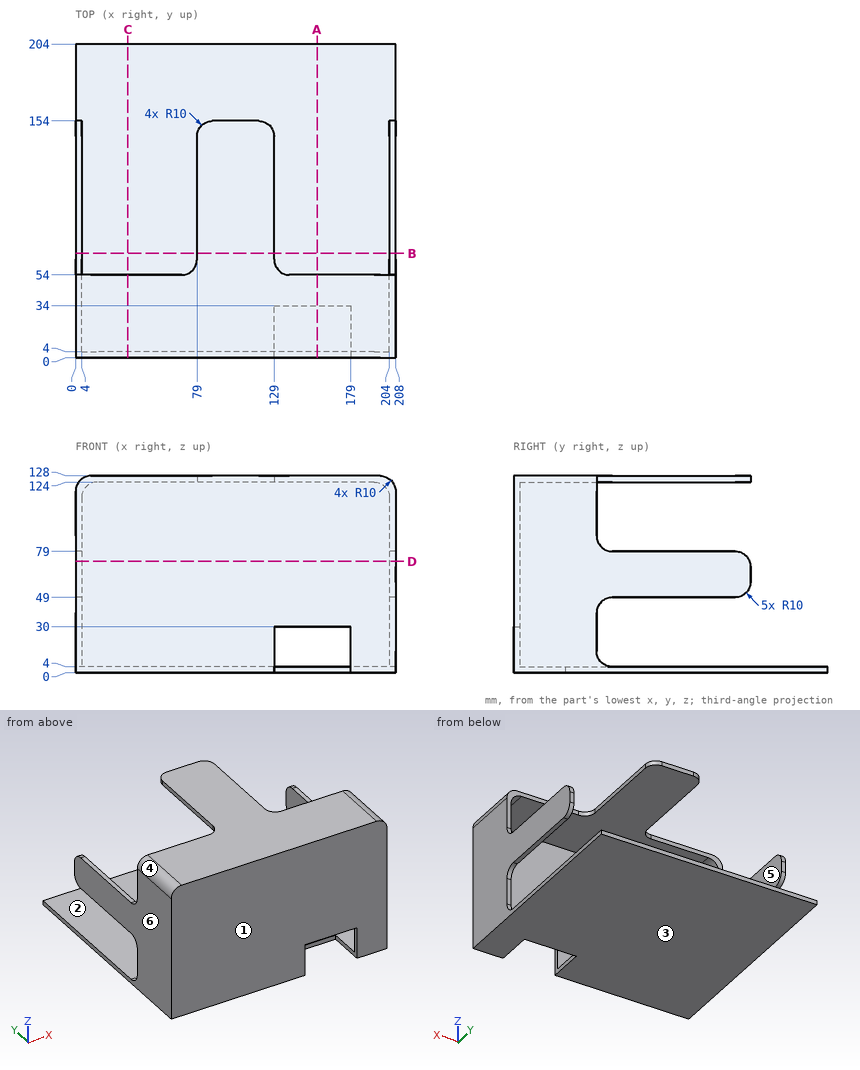
Part print with two shaded views. Sizes in mm from the minimum x, y, z corner. A direction names the side the tool comes from. Coordinates: 2 decimals unless noted, no trailing zeros. Write each loop counter-clockwise with the first axis right and the second up, starting at its lowest first coordinate (ties: lowest second). Pieces come first, ordered by that corner, then holes. Notation, with made-up numbers: (55, -29.5) - (99, -29.5) arc R26 ccw to (99, -0.5) - close; hole circle Ø7 at (48.25, 21). An arc over 180 degrees is marked (long way). Put each result on its own line as item: value.
1. Flat gauge pins, fed straight in: pin 1 Ø2 at (y, z) = (118, 126) entering from -X; pin 2 Ø2 at (x, z) = (111.5, 125.5) entering from +Y; pin 3 Ø12 at (x, z) = (159, 29.5) entering from +Y. Where does each tip first touch, or does it go through?
Final values:
pin 1: stops at x = 79
pin 2: stops at y = 154
pin 3: stops at y = 4
2. Band-saw the part on C-C (x = 34). Write the cut outline in (y, z).
Final values:
outline: (0, 0) - (204, 0) - (204, 4) - (4, 4) - (4, 124) - (54, 124) - (54, 128) - (0, 128) - close
3. Probe line 1 along Z through (x, y) = (51, 21.5); line 2 along X through (y, z) = (25, 106); line 3 along Z through (x, y) = (168, 21). List the from-to ranges inside material, lowest first. Write a range as [from, to].
Final values:
line 1: z = [0, 4], [124, 128]
line 2: x = [0, 4], [204, 208]
line 3: z = [124, 128]
4. Band-saw the part on B-B (y = 68). Write the cut outline in (x, z).
Final values:
outline: (0, 0) - (208, 0) - (208, 4) - (0, 4) - close; (0, 49) - (4, 49) - (4, 79) - (0, 79) - close; (79, 124) - (129, 124) - (129, 128) - (79, 128) - close; (204, 49) - (208, 49) - (208, 79) - (204, 79) - close
5. Two-plate mould, pull along Z, no slides. Class the marked faces 1, 2, 3 and 4: +Z half, -Z half, draft (parallel to the pull), parting line (faces both ways), or undercut.
Final values:
face 1: draft
face 2: undercut
face 3: -Z half
face 4: +Z half
6. Band-saw the part on A-A (x = 157). Write the cut outline in (y, z).
Final values:
outline: (0, 30) - (4, 30) - (4, 124) - (54, 124) - (54, 128) - (0, 128) - close; (34, 0) - (204, 0) - (204, 4) - (34, 4) - close
7. Band-saw the part on D-D (z = 72.5). Write the cut outline in (x, y).
Final values:
outline: (0, 0) - (208, 0) - (208, 153.37) - (204, 153.37) - (204, 4) - (4, 4) - (4, 153.37) - (0, 153.37) - close
8. 3-axis set-ups, long thin cutter, end or side, ignore diameter. For the marked faces 5 and 6: which of +Z, -Z, +X, -X, +Y, -Y reach the whole face in a straight line?
Final values:
face 5: +Y
face 6: +Z, -Z, -X, +Y, -Y
